Autodesk Inventor part; units mm, degrees
ref_plane "YZ Plane" through (0, 0, 0) normal (1, 0, 0) x (0, 1, 0)
ref_plane "XZ Plane" through (0, 0, 0) normal (0, 1, 0) x (-1, 0, 0)
ref_plane "XY Plane" through (0, 0, 0) normal (0, 0, 1) x (1, 0, 0)
sketch "Sketch1" plane through (0, 0, 0) normal (0, 0, 1) x (1, 0, 0)
  line L0 (0, 0) -> (80, 0)
  line L1 (80, 0) -> (80, -80)
  line L2 (80, -80) -> (0, -80)
  line L3 (0, -80) -> (0, 0)
  dimension "d0" = 80
  dimension "d1" = 80
extrude "Plate1" add sketch "Sketch1" against normal blind 2
sketch "Sketch2" plane through (78, 0, -2) normal (1, 0, 0) x (0, 1, 0)
  line L0 (-80, 0) -> (0, 0)
  line L1 (0, 0) -> (0, 80)
  line L2 (0, 80) -> (-80, 80)
  line L3 (-80, 80) -> (-80, 0)
edge flange "Flange1" height 80 angle 90 thickness 2 bend radius 2.5 thickness toward (1, 0, 0) relief round relief width 2 relief depth 1 edges at (80, -40, 0) wall of the first edge with corners at (78, -80, -2) (78, 0, -2) (78, 0, 78) (78, -80, 78)
bend "Bend1"
corner "Corner1"
sketch "Sketch3" plane through (0, 0, 0) normal (0, 0, 1) x (1, 0, 0)
  line L0 (75.5, 0) -> (0, 0)
  line L1 (75.5, -80) -> (75.5, 0)
  line L2 (0, 0) -> (75.5, -80) construction
  circle A0 centre (37.75, -40) radius 7.25
  dimension "d13" = 14.5
extrude "Extrusion1" cut sketch "Sketch3" against normal through all
equation "\"d2\" = Thickness"
equation "\"d3\" = BendReliefWidth"
equation "\"d4\" = BendReliefDepth"
equation "\"d5\" = MinimumRemnant"
equation "\"d6\" = TransitionRadius"
equation "\"d9\" = BendRadius"
equation "\"d10\" = CornerReliefSize"
equation "\"d11\" = GapSize"
equation "\"d12\" = JacobiRadiusSize"
equation "\"BendReliefWidth\" = Thickness"
equation "\"BendReliefDepth\" = 0.5 * Thickness"
equation "\"CornerReliefSize\" = 4 * Thickness"
equation "\"MinimumRemnant\" = 2 * Thickness"
equation "\"TransitionRadius\" = BendRadius"
equation "\"JacobiRadiusSize\" = BendRadius"
equation "\"GapSize\" = Thickness"
properties part number "ASY MSC Мостики уголок" material "Stainless Steel"
Part model, mm, in its own coordinate system. A direction names the side the tool comes from. Round coordinates to 2 decimals unless told otherwise and drop trailing zeros. Write each loop counter-clockwise with the first axis right and the second up, starting at its lowest first coordinate (ties: lowest second). Pieces come first, ordered by that corner, then holes.
Item 1: Which spindle directions (+Z, -Z, +X, -X, +Y, -Y) get a long thin tool onto all of the face, cutting with end or side? Do faces 5 (the flat face through (46, -39, 0)), 6 (the cylindrical face through (78.717, -39.44, -0.647)). Say none if no direction does.
Results:
face 5: +Z, -X, +Y, -Y
face 6: -Z, +X, +Y, -Y
Item 2: Cut at A-A, the plane y = -40. Give the cut face in (x, z), plus the area to 3 significant figures.
Results:
outline: (0, -2) - (30.5, -2) - (30.5, 0) - (0, 0) - close; (45, -2) - (75.5, -2) arc R4.5 ccw to (80, 2.5) - (80, 78) - (78, 78) - (78, 2.5) arc R2.5 cw to (75.5, 0) - (45, 0) - close
area: 284 mm2
Item 3: Drop flat-ended pins along their axis: pin 1 Ø2 at (y, z) = (-57.5, 25) entering from -X; pin 2 Ø13 at (x, y) = (37.75, -40) entering from -Z. Give the stop position or say it passes through.
Results:
pin 1: stops at x = 78
pin 2: passes through
Item 4: Cut at C-C, the plane y = -26. Give the cut face in (x, z).
Results:
outline: (0, -2) - (75.5, -2) arc R4.5 ccw to (80, 2.5) - (80, 78) - (78, 78) - (78, 2.5) arc R2.5 cw to (75.5, 0) - (0, 0) - close
Item 5: Cut at D-D, the plane z = 53.5. Give the cut face in (x, y), plus the area to 3 significant figures.
Results:
outline: (78, -80) - (80, -80) - (80, 0) - (78, 0) - close
area: 160 mm2
Item 6: Cut at B-B, the plane x = 37.75. Give the cut face in (y, z), plus the area to 3 significant figures.
Results:
outline: (-80, -2) - (-47.25, -2) - (-47.25, 0) - (-80, 0) - close; (-32.75, -2) - (0, -2) - (0, 0) - (-32.75, 0) - close
area: 131 mm2
Item 7: Two-plate mould, pull along Y, no slides. Class faces 1 (the flat face through (79, -80, 20)), 2 (the flat face through (79, 0, 20)), 3 (the flat face through (78, -39, 40)), 4 (the cylindrical face through (31.997, -44.412, -0.986)): +Y half, -Y half, draft (parallel to the pull), parting line (faces both ways), or undercut.
Results:
face 1: -Y half
face 2: +Y half
face 3: draft
face 4: undercut
Item 8: Probe L1, parallel to Y at x = 37.75, z = -1.05; L2, parallel to Z at x = 39, y = -25; L3, parallel to X at y = -35.5, z = 24. List the from-to ranges inside material, lowest first.
Results:
L1: y = -80 to -47.25, -32.75 to 0
L2: z = -2 to 0
L3: x = 78 to 80
